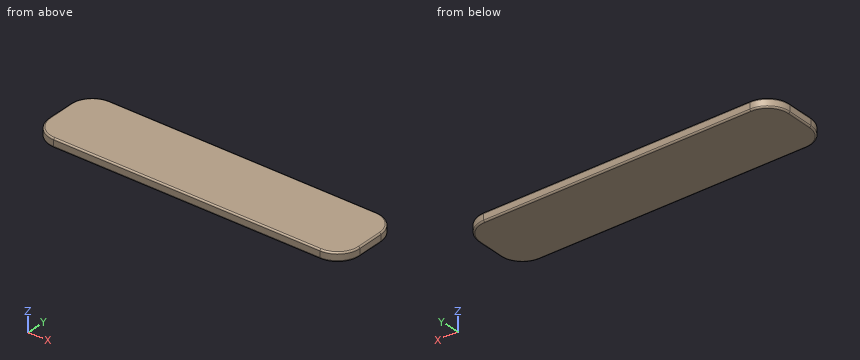
from build123d import *

# Parameters (mm, degrees)
F0_W     = 2100
F0_H     = 480
F1_DEPTH = 60
F2_R     = 150
F3_R     = 10


with BuildPart() as f1:
    # F0 (on Top) → F1 (new body)
    with BuildSketch(Plane.XY):
        Rectangle(F0_W, F0_H)
    extrude(amount=F1_DEPTH)

    # F2
    f2_edges = [f1.edges().sort_by_distance(p)[0] for p in [
        (-1050, -240, 30),
        (-1050, 240, 30),
        (1050, -240, 30),
        (1050, 240, 30),
    ]]
    fillet(f2_edges, radius=F2_R)

    # F3
    f3_edges = [f1.edges().sort_by_distance(p)[0] for p in [
        (0, -240, 60),
        (0, -240, 0),
    ]]
    fillet(f3_edges, radius=F3_R)


solid = f1.part
Geometry: final body of the model. Coordinates: model frame, mm. Coordinates: 2 decimals unless noted, no trailing zeros. Write each loop counter-clockwise with the first axis right and the second up, starting at its lowest first coordinate (ties: lowest second). Pieces come first, ordered by that corner, then holes. Notation, with made-up numbers: (4.5, 32.5) - (16.5, 32.5) arc R21 cw to (16.5, 40.5) - close; hole circle Ø10 at (-5.75, 54). An arc over 180 degrees is marked (long way). Return JSON: item names as keys, results as strings.
Item 1: Section query A-A (z = 22.5). Output: boundary loops of the cut face in (x, y).
Completed:
{"outline": "(-1050, -90) arc R150 ccw to (-900, -240) - (900, -240) arc R150 ccw to (1050, -90) - (1050, 90) arc R150 ccw to (900, 240) - (-900, 240) arc R150 ccw to (-1050, 90) - close"}
Item 2: Line query: L1, parallel to Y at x = -393.5, z = 51; L2, parallel to X at y = -3, z = 51; L3, parallel to X at y = 47, z = 56. Output: solid intervals per line, ascending.
Completed:
{"L1": "y = -239.95 to 239.95", "L2": "x = -1049.95 to 1049.95", "L3": "x = -1048 to 1048"}
Item 3: Pin query (flat end, axial travel): pin 1 Ø12 at (y, z) = (120, 21.5) entering from +X; pin 2 Ø3 at (x, z) = (-631.5, 7) entering from +Y. Return the tip coordinate at first contact, or that it passes through.
Completed:
{"pin 1": "stops at x = 1048.07", "pin 2": "stops at y = 239.89"}
